```python
from build123d import *

# Parameters (mm, degrees)
SKETCH_1_W           = 62.64
SKETCH_1_H           = 10
EXTRUDE_2_DEPTH      = 10
SKETCH_3_R           = 3
CUT_EXTRUDE_3_DEPTH  = 35.364842499
SKETCH_4_R           = 3
CUT_EXTRUDE_5_DEPTH  = 34.255712291
SKETCH_5_W           = 44.64
SKETCH_5_H           = 2
CUT_EXTRUDE_7_DEPTH  = 35.364842499
CUT_EXTRUDE_8_DEPTH  = 35.364842499
SKETCH_10_R          = 5
EXTRUDE_7_DEPTH      = 10
SKETCH_11_R          = 3
CUT_EXTRUDE_9_DEPTH  = 35.364842499
SKETCH_13_W          = 2
SKETCH_13_H          = 10
CUT_EXTRUDE_11_DEPTH = 54.814213736


with BuildPart() as part:
    # 草图1 → 凸台-拉伸2 (new body)
    with BuildSketch(Plane.XY):
        Rectangle(SKETCH_1_W, SKETCH_1_H)
    extrude(amount=EXTRUDE_2_DEPTH)

    # 草图3 → 切除-拉伸3 (cut, through all)
    with BuildSketch(Plane(origin=(0, 5, 0), x_dir=(1, 0, 0), z_dir=(0, 1, 0))):
        with BuildLine():
            ThreePointArc((31.32, -5), (29.855533906, -8.535533906), (26.32, -10))
            Line((26.32, -10), (31.32, -10))
            Line((31.32, -10), (31.32, -5))
        make_face()
        with BuildLine():
            Line((31.32, 0), (26.32, 0))
            ThreePointArc((26.32, 0), (29.855533906, -1.464466094), (31.32, -5))
            Line((31.32, -5), (31.32, 0))
        make_face()
        with Locations(Location((26.32, -5, 0), (0, 0, 270))):
            Circle(SKETCH_3_R)
    extrude(amount=-CUT_EXTRUDE_3_DEPTH, mode=Mode.SUBTRACT)

    # 草图4 → 切除-拉伸5 (cut, through all)
    with BuildSketch(Plane.XY.offset(10)):
        with BuildLine():
            ThreePointArc((-31.32, 0), (-29.855533906, 3.535533906), (-26.32, 5))
            Line((-26.32, 5), (-31.32, 5))
            Line((-31.32, 5), (-31.32, 0))
        make_face()
        with BuildLine():
            ThreePointArc((-26.32, -5), (-29.855533906, -3.535533906), (-31.32, 0))
            Line((-31.32, 0), (-31.32, -5))
            Line((-31.32, -5), (-26.32, -5))
        make_face()
        with Locations((-26.32, 0)):
            Circle(SKETCH_4_R)
    extrude(amount=-CUT_EXTRUDE_5_DEPTH, mode=Mode.SUBTRACT)

    # 草图5 → 切除-拉伸7 (cut, through all)
    with BuildSketch(Plane(origin=(0, 5, 0), x_dir=(1, 0, 0), z_dir=(0, 1, 0))):
        with Locations((1, -9)):
            Rectangle(SKETCH_5_W, SKETCH_5_H)
        with Locations((1, -1)):
            Rectangle(SKETCH_5_W, SKETCH_5_H)
    extrude(amount=-CUT_EXTRUDE_7_DEPTH, mode=Mode.SUBTRACT)

    # 草图6 → 切除-拉伸8 (cut, through all)
    with BuildSketch(Plane(origin=(0, 5, 0), x_dir=(1, 0, 0), z_dir=(0, 1, 0))):
        with BuildLine():
            Line((23.32, 0), (23.32, -1))
            ThreePointArc((23.32, -1), (24.73886117, -0.25658351), (26.32, 0))
            Line((26.32, 0), (23.32, 0))
        make_face()
        with BuildLine():
            ThreePointArc((26.32, -10), (24.73886117, -9.74341649), (23.32, -9))
            Line((23.32, -9), (23.32, -10))
            Line((23.32, -10), (26.32, -10))
        make_face()
    extrude(amount=-CUT_EXTRUDE_8_DEPTH, mode=Mode.SUBTRACT)

    # 草图10 → 凸台-拉伸7 (add)
    with BuildSketch(Plane(origin=(0, 5, 0), x_dir=(1, 0, 0), z_dir=(0, 1, 0))):
        with Locations((26.32, -5)):
            Circle(SKETCH_10_R)
    extrude(amount=-EXTRUDE_7_DEPTH)

    # 草图11 → 切除-拉伸9 (cut, through all)
    with BuildSketch(Plane(origin=(0, 5, 0), x_dir=(1, 0, 0), z_dir=(0, 1, 0))):
        with Locations(Location((26.32, -5, 0), (0, 0, 270))):
            Circle(SKETCH_11_R)
    extrude(amount=-CUT_EXTRUDE_9_DEPTH, mode=Mode.SUBTRACT)

    # 草图13 → 切除-拉伸11 (cut, through all)
    with BuildSketch(Plane(origin=(-21.32, 0, 0), x_dir=(0, 0, -1), z_dir=(1, 0, 0))):
        with Locations((-9, 0)):
            Rectangle(SKETCH_13_W, SKETCH_13_H)
        with Locations((-1, 0)):
            Rectangle(SKETCH_13_W, SKETCH_13_H)
    extrude(amount=-CUT_EXTRUDE_11_DEPTH, mode=Mode.SUBTRACT)


solid = part.part
```
For this review, take the finished solid that the model builds, in its own axes (mm). A direction names the side the tool comes from. Coordinates: 2 decimals unless noted, no trailing zeros. Order: outer loops, then holes, each group sorted by start corner. A loop starts at its lowest first (then second) coordinate and runs counter-clockwise, first axis right, second up. Notation, with made-up numbers: (34, 64.5) - (58, 64.5) arc R20 ccw to (58, 78.5) - close; hole circle Ø10 at (82, 63). An arc over 180 degrees is marked (long way). Answer as a JSON object with one key per item and string values. Group by question number.
1. We need section B-B on y = -3.75. State the section outline as (x, z) points, then the cut area to 3 significant figures.
2. Clearance check with flat-ended pins moving along their axes: P1, Ø3, axis at x = -4, y = 1.5, coming from the -Z side; P2, Ø1, axis at x = 23, y = 2.5, coming from the -Z side; P3, Ø6, axis at y = 3, z = 1, coming from the -X side. State where each tip first meets the part, or that it passes through.
3. We need section A-A on z = 4.25. State the section outline as (x, y) points, then the cut area to 3 significant figures.
4. For probe 1 along Y at (x, z) = (-26.32, 6.2); probe 2 along X at (y, z) = (2.75, 5); probe 3 along X at (y, z) = (2.5, 2.75), list the stretches that pass through material, from the lowest coordinate up.
5. We need section C-C on x = 21. State the section outline as (y, z) points, then the cut area to 3 significant figures.
6. We need section D-D on y = 4.25. State the section outline as (x, z) points, then the cut area to 3 significant figures.
7. The part is to be moulded in two halves that separate along Y. For faces 1 (the flat face through (2, -5, 5)), 2 (the cylindrical face through (-23.55, -1.15, 5.04)), 3 (the flat face through (2, 5, 5)), 4 (the flat face through (-4, 0, 2)), say which applies: pulls with the +Y half, pulls with the -Y half, needs draft (parallel to the pull), parting line crosses it, or undercut.
8. For faces 5 (the flat face through (-5, 0, 8)), 6 (the cylindrical face through (23.39, 0.07, 4.35)), list the 3-axis set-ups (+Z, -Z, +X, -X, +Y, -Y) from which the entire face can be reached by the end or side of a thin tool; tool diameter is ignored.
Final values:
{
 "1": {"outline": "(-29.63, 2) - (22.32, 2) arc R5 ccw (long way) to (22.32, 8) - (-29.63, 8) - close; hole circle Ø6 at (26.32, 5)", "area": "358 mm²"},
 "2": {"P1": "z = 2", "P2": "z = 0.87", "P3": "x = -31.32"},
 "3": {"outline": "(-26.32, -5) - (23.42, -5) - (23.42, 5) - (-26.32, 5) arc R5 ccw to start; (29.22, -5) - (31.26, -5) - (31.26, 5) - (29.22, 5) - close; hole circle Ø6 at (-26.32, 0)", "area": "529 mm²"},
 "4": {"probe 1": "-5 to -3, 3 to 5", "probe 2": "-30.5 to -27.52, -25.12 to 23.32, 29.32 to 31.32", "probe 3": "-30.65 to -27.98, -24.66 to 24.34, 28.3 to 30.79"},
 "5": {"outline": "(-5, 2) - (5, 2) - (5, 8) - (-5, 8) - close", "area": "60.0 mm²"},
 "6": {"outline": "(-28.95, 2) - (22.32, 2) arc R5 ccw (long way) to (22.32, 8) - (-28.95, 8) - close; hole circle Ø6 at (26.32, 5)", "area": "354 mm²"},
 "7": {"face 1": "pulls with the -Y half", "face 2": "undercut", "face 3": "pulls with the +Y half", "face 4": "needs draft"},
 "8": {"face 5": "+Z, -X, +Y, -Y", "face 6": "+Y, -Y"}
}
